Geometry check sheet. Reference: the model listing, model coordinates, mm. A direction names the side the tool comes from. Give positions to 0.01 mm unless a question says otherwise; leave off trailing zeros. Loops run counter-clockwise (first coordinate to the right, second up) from the corner with the lowest first, then second, coordinate; pieces in that order, holes last. Notation, with made-up numbers: (-8.5, -10.5) - (16.5, -10.5) arc R19 cw to (16.5, -5.5) - close; hole circle Ø8 at (-19.5, 89). An arc over 180 degrees is marked (long way). Use a Markdown table: item, result. Add a question column.
1. Cross-section at C-C on z = 5.75. Enter the section's corners in (x, y).
2. Cross-section at A-A on x = -9.5. Enter the section's corners in (y, z), and give its area (3 significant figures).
3. Set-up check for faces 1 (the flat face through (-9, 1, 8)), 2 (the cylindrical face through (0.9, 25.74, 2.86)), 3 (the cylindrical face through (1, -3, 0)), 4 (the flat face through (-9, -1, 6)), 5 (the flat face through (4, -1, 0)): record each of +Z, -Z, +X, -X, +Y, -Y from which the full face is reachable in a straight line by a thin tool's end or side.
4. Depth check by flat-ended pin: P1, Ø10, axis at x = -4.5, y = 12.5, coming from the -Z side; P2, Ø8, axis at x = -6, z = -7, coming from the -Y side; P3, Ø1.5, axis at x = -9.5, z = 6, coming from the +Y side; P4, Ø10, axis at x = -1.5, y = 30.5, coming from the +Z side. Enter the tip coordinate at first touch or a pass-through.
5. Cross-section at D-D on x = 0. Enter the section's corners in (y, z), and give its area (3 significant figures).
6. Draft check along X on faces 6 (the flat face through (-9, 1, -4)), 7 (the cylindrical face through (-1, 31, 0)), 8 (the flat face through (-7.5, 1, -7)), 9 (the flat face through (-10.5, 1, 6)). Enter one of: pulls with the +X half, pulls with the -X half, needs draft (parallel to the pull), parting line crosses it, or undercut.
7. Material ranges on L1, parallel to X at y = 10.5, z = -4.5; L2, parallel to Y at x = -4.25, z = 4; L3, parallel to Z at x = 6, y = 21, recorded low to high.
8. Cross-section at B-B on y = 1. Enter the section's corners in (x, z), and give its area (3 significant figures).
from build123d import *

# Parameters (mm, degrees)
SKETCH_1_R            = 10
EXTRUDE_1_DEPTH       = 25
CUT_EXTRUDE_2_1_REACH = 30.723
SKETCH_2_W            = 2.5
SKETCH_2_H            = 20
SKETCH_3_R            = 3
EXTRUDE_2_DEPTH       = 1.5
EXTRUDE_START         = -1.5
SKETCH_4_R            = 1
EXTRUDE_3_DEPTH       = 10
EXTRUDE_START_2       = -25
EXTRUDE_4_DEPTH       = 27.3
EXTRUDE_START_3       = 1
SKETCH_6_R            = 1
EXTRUDE_5_DEPTH       = 1
SKETCH_7_W            = 4
SKETCH_7_H            = 4
EXTRUDE_6_DEPTH       = 3


with BuildPart() as part:
    # 草图1 → 圆柱凸台-拉伸1 (new body)
    with BuildSketch(Plane(origin=(0, 0, 0), x_dir=(1, 0, 0), z_dir=(0, 1, 0))):
        with Locations(Location((0, 0, 0), (0, 0, 270))):
            Circle(SKETCH_1_R)
    extrude(amount=EXTRUDE_1_DEPTH)

    # 草图2 → 2边切除切除-拉伸1 (cut, up to next)
    with BuildSketch(Plane.XZ, mode=Mode.PRIVATE) as cut_extrude_2_1_sk1:
        with Locations((-8.75, 0)):
            Rectangle(SKETCH_2_W, SKETCH_2_H)
    cut_extrude_2_1_tool1 = extrude(cut_extrude_2_1_sk1.sketch, amount=-CUT_EXTRUDE_2_1_REACH, mode=Mode.PRIVATE) & part.part
    # 草图2 → 2边切除切除-拉伸1 (cut, up to next)
    with BuildSketch(Plane.XZ, mode=Mode.PRIVATE) as cut_extrude_2_1_sk2:
        with Locations((8.75, 0)):
            Rectangle(SKETCH_2_W, SKETCH_2_H)
    cut_extrude_2_1_tool2 = extrude(cut_extrude_2_1_sk2.sketch, amount=-CUT_EXTRUDE_2_1_REACH, mode=Mode.PRIVATE) & part.part
    add(cut_extrude_2_1_tool1.solids().sort_by_distance((-8.75, 0, 0))[0], mode=Mode.SUBTRACT)
    add(cut_extrude_2_1_tool2.solids().sort_by_distance((8.75, 0, 0))[0], mode=Mode.SUBTRACT)

    # 草图3 → 前转凸台-拉伸2 (add)
    with BuildSketch(Plane(origin=(0, 25, 0), x_dir=(1, 0, 0), z_dir=(0, 1, 0))):
        with Locations(Location((0, 0, 0), (0, 0, 270))):
            Circle(SKETCH_3_R)
    extrude(amount=EXTRUDE_2_DEPTH)

    # 草图4 → 前转杆凸台-拉伸3 (add)
    with BuildSketch(Plane(origin=(0, 26.5, 0), x_dir=(1, 0, 0), z_dir=(0, 1, 0)).offset(EXTRUDE_START)):
        with Locations(Location((0, 0, 0), (0, 0, 270))):
            Circle(SKETCH_4_R)
    extrude(amount=EXTRUDE_3_DEPTH)

    # 草图5 → 后转凸台-拉伸4 (add)
    with BuildSketch(Plane.XZ.offset(EXTRUDE_START_2)):
        with BuildLine():
            Line((4, 3), (4, -3))
            ThreePointArc((4, -3), (-5, 0), (4, 3))
        make_face()
    extrude(amount=EXTRUDE_4_DEPTH)

    # 草图6 → 后转杆凸台-拉伸5 (add)
    with BuildSketch(Plane.XZ.offset(2.3).offset(EXTRUDE_START_3)):
        with Locations(Location((0, 0, 0), (0, 0, 90))):
            Circle(SKETCH_6_R)
    extrude(amount=-EXTRUDE_5_DEPTH)

    # 草图7 → 引线凸台-拉伸6 (add)
    with BuildSketch(Plane.ZY.offset(7.5)):
        with Locations((-6, 1)):
            Rectangle(SKETCH_7_W, SKETCH_7_H)
        with Locations((6, 1)):
            Rectangle(SKETCH_7_W, SKETCH_7_H)
    extrude(amount=EXTRUDE_6_DEPTH)


solid = part.part
Values found:
| question | item | result |
|---|---|---|
| 1 | outline | (-10.5, -1) - (-7.5, -1) - (-7.5, 0) - (7.5, 0) - (7.5, 25) - (-7.5, 25) - (-7.5, 3) - (-10.5, 3) - close |
| 2 | outline | (-1, -8) - (3, -8) - (3, -4) - (-1, -4) - close; (-1, 4) - (3, 4) - (3, 8) - (-1, 8) - close |
| 2 | area | 32.0 mm2 |
| 3 | face 1 | +Z, -X, +Y, -Y |
| 3 | face 2 | +Y |
| 3 | face 3 | -Y |
| 3 | face 4 | +Z, -Z, -X, -Y |
| 3 | face 5 | +Z, -Z, +X, -Y |
| 4 | P1 | stops at z = -10 |
| 4 | P2 | stops at y = -1 |
| 4 | P3 | stops at y = 3 |
| 4 | P4 | stops at z = 3 |
| 5 | outline | (-3.3, -1) - (-2.3, -1) - (-2.3, -5) - (0, -5) - (0, -10) - (25, -10) - (25, -3) - (26.5, -3) - (26.5, -1) - (35, -1) - (35, 1) - (26.5, 1) - (26.5, 3) - (25, 3) - (25, 10) - (0, 10) - (0, 5) - (-2.3, 5) - (-2.3, 1) - (-3.3, 1) - close |
| 5 | area | 551 mm2 |
| 6 | face 6 | needs draft |
| 6 | face 7 | parting line crosses it |
| 6 | face 8 | undercut |
| 6 | face 9 | pulls with the -X half |
| 7 | L1 | x = -7.5 to 7.5 |
| 7 | L2 | y = 0 to 25 |
| 7 | L3 | z = -8 to 8 |
| 8 | outline | (-10.5, -8) - (-7.5, -8) - (-7.5, -6.61) arc R10 ccw to (7.5, -6.61) - (7.5, 6.61) arc R10 ccw to (-7.5, 6.61) - (-7.5, 8) - (-10.5, 8) - (-10.5, 4) - (-7.5, 4) - (-7.5, -4) - (-10.5, -4) - close |
| 8 | area | 293 mm2 |
